Input: part model. Units: mm. Frame: model coordinates. Give positions to 0.01 mm unless a question says otherwise; leave off trailing zeros. Loops run counter-clockwise (first coordinate to the right, second up) from the corner with the lowest first, then second, coordinate; pieces in that order, holes last. Notation, with made-up numbers: (1.5, 72) -> (43.5, 72) arc R33 cw to (43.5, 103) -> close; hole circle Ø10 at (20.25, -25). An arc over 180 degrees is marked (long way). Answer as a JSON object with one key per item and string values.
```python
from build123d import *

# Parameters (mm, degrees)
SKETCH_1_W      = 149.5
SKETCH_1_H      = 149.5
EXTRUDE_1_DEPTH = 3
SKETCH_2_W      = 165
SKETCH_2_H      = 165
EXTRUDE_2_DEPTH = 2
FILLET_1_R      = 1
FILLET_2_R      = 2


with BuildPart() as part:
    # 草图1 → 凸台-拉伸1 (new body)
    with BuildSketch(Plane.XY):
        Rectangle(SKETCH_1_W, SKETCH_1_H)
    extrude(amount=EXTRUDE_1_DEPTH)

    # 草图2 → 凸台-拉伸2 (add)
    with BuildSketch(Plane.XY.offset(3)):
        Rectangle(SKETCH_2_W, SKETCH_2_H)
    extrude(amount=EXTRUDE_2_DEPTH)

    # 圆角1
    fillet_1_edges = [part.edges().sort_by_distance(p)[0] for p in [
        (74.75, -74.75, 1.5),
        (-74.75, -74.75, 1.5),
        (-74.75, 74.75, 1.5),
        (74.75, 74.75, 1.5),
    ]]
    fillet(fillet_1_edges, radius=FILLET_1_R)

    # 圆角2
    fillet_2_edges = [part.edges().sort_by_distance(p)[0] for p in [
        (0, -82.5, 5),
        (-82.5, 0, 5),
        (0, 82.5, 5),
        (82.5, 0, 5),
    ]]
    fillet(fillet_2_edges, radius=FILLET_2_R - 0.0001)  # a hair under: the kernel refuses the full size


solid = part.part
```
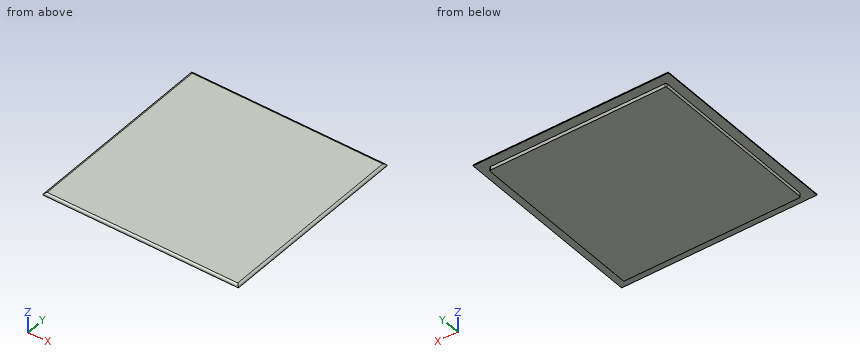
Q1. Pin query (flat end, axial travel): pin 1 (1.5 mm diameter, centred on y = 11, z = 1.5, fed in from -X); pin 2 (0.9 mm diameter, centred on y = 30, z = 1.5, fed in from +X). Return the tip coordinate at first contact, or that it passes through.
Evaluation:
{"pin 1": "stops at x = -74.75", "pin 2": "stops at x = 74.75"}
Q2. Section B-B, the plane z = 0.9. Return the cut outline in (x, y), then the cut area to 3 significant figures.
Evaluation:
{"outline": "(-74.75, -73.75) arc R1 ccw to (-73.75, -74.75) -> (73.75, -74.75) arc R1 ccw to (74.75, -73.75) -> (74.75, 73.75) arc R1 ccw to (73.75, 74.75) -> (-73.75, 74.75) arc R1 ccw to (-74.75, 73.75) -> close", "area": "22,300 mm2"}
Q3. Ray query, line 1 along X through (y, z) = (-53, 1.95); line 2 along X through (y, z) = (60, 3.1). Return the intervals inside material, ascending.
Evaluation:
{"line 1": "x = -74.75 to 74.75", "line 2": "x = -82.5 to 82.5"}
